Read the model definition and answer for the solid it produces. Units are mm, in the model's axes. A direction names the side the tool comes from. Give positions to 0.01 mm unless a question says otherwise; leave off trailing zeros. Loops run counter-clockwise (first coordinate to the right, second up) from the corner with the lowest first, then second, coordinate; pieces in that order, holes last. Notation, with made-up numbers: (60.25, 68) - (88.25, 68) arc R14 ccw to (88.25, 82) - close; hole circle Ø7 at (22, 68). An arc over 180 degrees is marked (long way). Put each result on its own line as item: value. Start each with the question number.
1. A cutting plane is placed at C-C, the plane x = -26. Determine the outline of the cut face in (y, z).
2. A cutting plane is placed at B-B, the plane x = 37.5. Determine the outline of the cut face in (y, z).
3. Given pin 1 Ø4.5 at (x, y) = (1, 2) entering from +Z; pin 2 Ø4 at (x, z) = (-3.5, 3) entering from -Y; pin 3 Ø2.5 at (x, y) = (37.5, -15.5) entering from -Z; pin 4 Ø0.6 at (x, z) = (-14, 6.5) entering from +Y, each flat-ended and moving along its own axis, determine where each tip first touches the part or whether it passes through.
4. For faces 4 (the flat face through (35, 0, 3)), 5 (the flat face through (0, 0, 6.5)), 6 (the flat face through (0, 12, 3)), determine the directions among +Z, -Z, +X, -X, +Y, -Y from which every point of the face is accessible in a straight line to the end or side of a thin tool.
5. A cutting plane is placed at D-D, the plane y = -0.5. Determine the outline of the cut face in (x, z), plus the area to 4 significant figures.
6. A cutting plane is placed at A-A, the plane y = 15.5. Determine the outline of the cut face in (x, z), plus the area to 3 significant figures.
7. Consider L1, parallel to Y at x = -37.5, z = -1.1; L2, parallel to X at y = -8.5, z = 5.5; L3, parallel to Y at x = 17, z = 3.5. Determine where each line is inside the solid, lowest interval first. Write a range as from..to.
8. For a pull along Y with two mould halves and no side action, classify faces 1 (the cylindrical face through (38.7, -16.4, -0.8)), 2 (the flat face through (40, 0, -1)), 3 (the flat face through (-1, 18, -1)) as released by +Y, released by -Y, zero draft, split by the parting line, or undercut.
```python
from build123d import *

# Parameters (mm, degrees)
SKETCH1_W           = 80
SKETCH1_H           = 36
BASE_FLANGE1_DEPTH  = 1.5
SKETCH6_W           = 70
SKETCH6_H           = 24
BOSS_EXTRUDE1_DEPTH = 7
SKETCH7_W           = 65
SKETCH7_H           = 15
CUT_EXTRUDE1_DEPTH  = 0.5
CUT_EXTRUDE2_DEPTH  = 0.5
CUT_EXTRUDE3_REACH  = 46.679
SKETCH9_R           = 1.5


# Sheet-metal steps are written as plain solids
with BuildPart() as part:
    # Sketch1 → Base-Flange1 (new body)
    with BuildSketch(Plane.XY):
        Rectangle(SKETCH1_W, SKETCH1_H)
    extrude(amount=-BASE_FLANGE1_DEPTH)

    # Sketch6 → Boss-Extrude1 (add)
    with BuildSketch(Plane.XY):
        Rectangle(SKETCH6_W, SKETCH6_H)
    extrude(amount=BOSS_EXTRUDE1_DEPTH)

    # Sketch7 → Cut-Extrude1 (cut)
    with BuildSketch(Plane.XY.offset(7)):
        Rectangle(SKETCH7_W, SKETCH7_H)
    extrude(amount=-CUT_EXTRUDE1_DEPTH, mode=Mode.SUBTRACT)

    # Sketch8 → Cut-Extrude2 (cut)
    with BuildSketch(Plane.XY.offset(7)):
        with BuildLine():
            Line((32, 9.25), (-32, 9.25))
            ThreePointArc((-32, 9.25), (-32.5, 9.75), (-32, 10.25))
            Line((-32, 10.25), (32, 10.25))
            ThreePointArc((32, 10.25), (32.5, 9.75), (32, 9.25))
        make_face()
        with BuildLine():
            Line((32, -9.25), (-32, -9.25))
            ThreePointArc((-32, -9.25), (-32.5, -9.75), (-32, -10.25))
            Line((-32, -10.25), (32, -10.25))
            ThreePointArc((32, -10.25), (32.5, -9.75), (32, -9.25))
        make_face()
    extrude(amount=-CUT_EXTRUDE2_DEPTH, mode=Mode.SUBTRACT)

    # Sketch9 → Cut-Extrude3 (cut, up to next)
    with BuildSketch(Plane(origin=(0, 0, -1.5), x_dir=(-1, 0, 0), z_dir=(0, 0, -1)), mode=Mode.PRIVATE) as cut_extrude3_sk1:
        with Locations((-37.5, 15.5)):
            Circle(SKETCH9_R)
    cut_extrude3_tool1 = extrude(cut_extrude3_sk1.sketch, amount=-CUT_EXTRUDE3_REACH, mode=Mode.PRIVATE) & part.part
    # Sketch9 → Cut-Extrude3 (cut, up to next)
    with BuildSketch(Plane(origin=(0, 0, -1.5), x_dir=(-1, 0, 0), z_dir=(0, 0, -1)), mode=Mode.PRIVATE) as cut_extrude3_sk2:
        with Locations((-37.5, -15.5)):
            Circle(SKETCH9_R)
    cut_extrude3_tool2 = extrude(cut_extrude3_sk2.sketch, amount=-CUT_EXTRUDE3_REACH, mode=Mode.PRIVATE) & part.part
    # Sketch9 → Cut-Extrude3 (cut, up to next)
    with BuildSketch(Plane(origin=(0, 0, -1.5), x_dir=(-1, 0, 0), z_dir=(0, 0, -1)), mode=Mode.PRIVATE) as cut_extrude3_sk3:
        with Locations((37.5, 15.5)):
            Circle(SKETCH9_R)
    cut_extrude3_tool3 = extrude(cut_extrude3_sk3.sketch, amount=-CUT_EXTRUDE3_REACH, mode=Mode.PRIVATE) & part.part
    # Sketch9 → Cut-Extrude3 (cut, up to next)
    with BuildSketch(Plane(origin=(0, 0, -1.5), x_dir=(-1, 0, 0), z_dir=(0, 0, -1)), mode=Mode.PRIVATE) as cut_extrude3_sk4:
        with Locations((37.5, -15.5)):
            Circle(SKETCH9_R)
    cut_extrude3_tool4 = extrude(cut_extrude3_sk4.sketch, amount=-CUT_EXTRUDE3_REACH, mode=Mode.PRIVATE) & part.part
    add(cut_extrude3_tool1.solids().sort_by_distance((37.5, 15.5, -1.5))[0], mode=Mode.SUBTRACT)
    add(cut_extrude3_tool2.solids().sort_by_distance((37.5, -15.5, -1.5))[0], mode=Mode.SUBTRACT)
    add(cut_extrude3_tool3.solids().sort_by_distance((-37.5, 15.5, -1.5))[0], mode=Mode.SUBTRACT)
    add(cut_extrude3_tool4.solids().sort_by_distance((-37.5, -15.5, -1.5))[0], mode=Mode.SUBTRACT)


solid = part.part
```
Return value:
1. outline: (-18, -1.5) - (18, -1.5) - (18, 0) - (12, 0) - (12, 7) - (10.25, 7) - (10.25, 6.5) - (9.25, 6.5) - (9.25, 7) - (7.5, 7) - (7.5, 6.5) - (-7.5, 6.5) - (-7.5, 7) - (-9.25, 7) - (-9.25, 6.5) - (-10.25, 6.5) - (-10.25, 7) - (-12, 7) - (-12, 0) - (-18, 0) - close
2. outline: (-18, -1.5) - (-17, -1.5) - (-17, 0) - (-18, 0) - close; (-14, -1.5) - (14, -1.5) - (14, 0) - (-14, 0) - close; (17, -1.5) - (18, -1.5) - (18, 0) - (17, 0) - close
3. pin 1: stops at z = 6.5
3. pin 2: stops at y = -12
3. pin 3: passes through
3. pin 4: stops at y = 12
4. face 4: +Z, +X, +Y, -Y
4. face 5: +Z
4. face 6: +Z, +X, -X, +Y
5. outline: (-40, -1.5) - (40, -1.5) - (40, 0) - (35, 0) - (35, 7) - (32.5, 7) - (32.5, 6.5) - (-32.5, 6.5) - (-32.5, 7) - (-35, 7) - (-35, 0) - (-40, 0) - close
5. area: 577.5 mm2
6. outline: (-40, -1.5) - (-39, -1.5) - (-39, 0) - (-40, 0) - close; (-36, -1.5) - (36, -1.5) - (36, 0) - (-36, 0) - close; (39, -1.5) - (40, -1.5) - (40, 0) - (39, 0) - close
6. area: 111 mm2
7. L1: y = -18..-17, -14..14, 17..18
7. L2: x = -35..35
7. L3: y = -12..12
8. face 1: undercut
8. face 2: zero draft
8. face 3: released by +Y
